The listing builds one solid part. Answer for the finished solid, in the listing's coordinates (mm). Face numbers are marked on the shaded views. A direction names the side the tool comes from. Coordinates: 2 decimals unless noted, no trailing zeros. Loops run counter-clockwise (first coordinate to the right, second up) from the corner with the lowest first, then second, coordinate; pieces in that order, holes last. Notation, with made-up numbers: (66, 87.5) -> (92, 87.5) arc R20 cw to (92, 124.5) -> close; hole circle Ø1 at (-6.5, 33.25). An arc over 180 degrees is marked (long way). Answer in a Markdown table with one row per item.
```python
from build123d import *

# Parameters (mm, degrees)
F0_W     = 148
F0_H     = 12
F1_DEPTH = 39
F2_DEPTH = 29
F3_W     = 123
F3_H     = 12
F3_W_2   = 15
F3_W_3   = 10
F4_DEPTH = 4
F5_R     = 4.5
F6_DEPTH = 36


with BuildPart() as f1:
    # F0 (on Front) → F1 (new body)
    with BuildSketch(Plane.XZ):
        with Locations((0, 12)):
            Rectangle(F0_W, F0_H)
        with Locations((0, -12)):
            Rectangle(F0_W, F0_H)
        Rectangle(F0_W, F0_H)
    extrude(amount=F1_DEPTH)

    # F0 (on Front) → F2 (cut)
    with BuildSketch(Plane.XZ):
        Rectangle(F0_W, F0_H)
    extrude(amount=F2_DEPTH, mode=Mode.SUBTRACT)

    # F3 (on face) → F4 (cut)
    with BuildSketch(Plane.XZ.offset(39)):
        with Locations((12.5, 0)):
            Rectangle(F3_W, F3_H)
        with Locations((-56.5, 0)):
            Rectangle(F3_W_2, F3_H)
        with Locations((-69, 0)):
            Rectangle(F3_W_3, F3_H)
        with Locations((-56.5, 12)):
            Rectangle(F3_W_2, F3_H)
        with Locations((-56.5, -12)):
            Rectangle(F3_W_2, F3_H)
    extrude(amount=-F4_DEPTH, mode=Mode.SUBTRACT)

    # F5 (on face) → F6 (cut)
    with BuildSketch(Plane.XY.offset(18)):
        with Locations((64, -29)):
            Circle(F5_R)
    extrude(amount=-F6_DEPTH, mode=Mode.SUBTRACT)


solid = f1.part
```
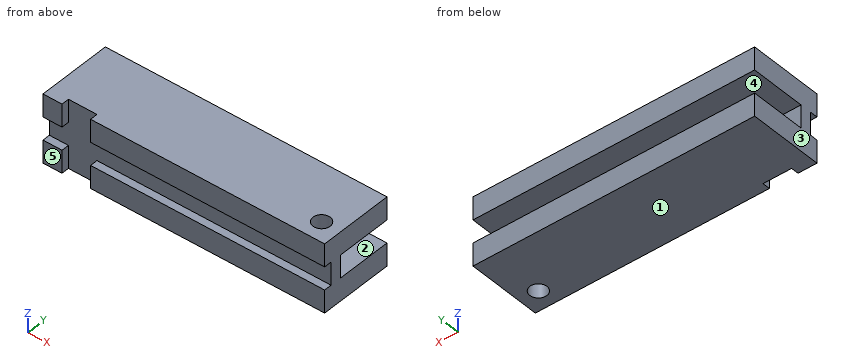
Item 1: Determine the mould class of the marked faces 1, 2 and 3 for opening direction Z: +Z half, -Z half, draft (parallel to the pull), parting line (faces both ways), or undercut.
Findings below:
| item | result |
|---|---|
| face 1 | -Z half |
| face 2 | undercut |
| face 3 | draft |
Item 2: Flat-ended cylindrical pins translate along their axes: pin 1 Ø6 at (x, z) = (-5.5, 1.5) entering from +Y; pin 2 Ø13 at (x, z) = (-15, -1.5) entering from +Y. Find the tip coordinate at first contact, or state that the pin passes through.
Findings below:
| item | result |
|---|---|
| pin 1 | stops at y = -29 |
| pin 2 | stops at y = 0 |
Item 3: A cutting plane is placed at A-A, the plane x = 64. Determine the outline of the cut face in (y, z).
Findings below:
| item | result |
|---|---|
| outline | (-39, -18) -> (-33.5, -18) -> (-33.5, 18) -> (-39, 18) -> (-39, 6) -> (-35, 6) -> (-35, -6) -> (-39, -6) -> close; (-24.5, -18) -> (0, -18) -> (0, -6) -> (-24.5, -6) -> close; (-24.5, 6) -> (0, 6) -> (0, 18) -> (-24.5, 18) -> close |
Item 4: A cutting plane is placed at C-C, the plane y = -16.5. Determine the outline of the cut face in (x, z).
Findings below:
| item | result |
|---|---|
| outline | (-74, -18) -> (74, -18) -> (74, -6) -> (-74, -6) -> close; (-74, 6) -> (74, 6) -> (74, 18) -> (-74, 18) -> close |
Item 5: A cutting plane is placed at B-B, the plane z = -8.5. Determine the outline of the cut face in (x, y), plus the area to 3 significant figures.
Findings below:
| item | result |
|---|---|
| outline | (-74, -39) -> (-64, -39) -> (-64, -35) -> (-49, -35) -> (-49, -39) -> (74, -39) -> (74, 0) -> (-74, 0) -> close; hole circle Ø9 at (64, -29) |
| area | 5,650 mm2 |
Item 6: Find the intervals of material crossed by probe 1 along Z at (x, y) = (-45, -2.5); probe 2 along X at (y, z) = (-28.5, 13); probe 3 along Y at (x, z) = (64, -9), in increasing order.
Findings below:
| item | result |
|---|---|
| probe 1 | z = -18 to -6, 6 to 18 |
| probe 2 | x = -74 to 59.53, 68.47 to 74 |
| probe 3 | y = -39 to -33.5, -24.5 to 0 |
Item 7: A cutting plane is placed at D-D, the plane x = -1.5. Determine the outline of the cut face in (y, z).
Findings below:
| item | result |
|---|---|
| outline | (-39, -18) -> (0, -18) -> (0, -6) -> (-29, -6) -> (-29, 6) -> (0, 6) -> (0, 18) -> (-39, 18) -> (-39, 6) -> (-35, 6) -> (-35, -6) -> (-39, -6) -> close |
Item 8: A tool of negligible diameter and unlimited length cuts with its end or side. For the marked faces 4 and 5, from which of +Z, -Z, +X, -X, +Y, -Y can it reach the whole face along a straight path? Write none if from no direction.
Findings below:
| item | result |
|---|---|
| face 4 | +X, -X, +Y |
| face 5 | +Z, -Z, +X, -X, -Y |
